Geometry: final body of the model. Coordinates: model frame, mm. Round coordinates to 2 decimals unless told otherwise and drop trailing zeros. Loops run counter-clockwise (first coordinate to the right, second up) from the corner with the lowest first, then second, coordinate; pieces in that order, holes last. Notation, with made-up numbers: (-30.5, 29.25) - (26.5, 29.25) arc R20 ccw to (26.5, 47.25) - close; hole circle Ø11 at (18, 40). An arc over 180 degrees is marked (long way). Answer as a JSON object with one key per item and string values. Group by question number.
Item 1: Section C-C (z = 1). Count the separate pieces of the cut face and the enclosed holes in it, plus the area to 3 significant figures.
Item 2: First-contact query: pin 1 (2.5 mm diameter, centred on x = 35.47, y = 25.41, fed in from -Z); pin 2 (12 mm diameter, centred on x = 11, y = -12.5, fed in from -Z). Flat tips, straight axial feed; report the tip coordinate or a pass-through.
Item 3: Section A-A (y = 2). Return the cut outline in (x, z).
Item 4: Line query: line 1 (X direction, y = 2, z = 0.7); line 2 (X direction, y = 16.5, z = 0.4); line 3 (Y direction, x = 35, z = 1.45). Output: solid intervals per line, ascending.
Item 5: Section B-B (x = 15.5). Return the cut outline in (y, z), plus the area to 3 significant figures.
```python
from build123d import *

# Parameters (mm, degrees)
SKETCH1_W                        = 39.2
SKETCH1_H                        = 58.746225757
BASE_DEPTH                       = 1.5
FRONT_FILLET_R                   = 5
BOLT_HOLE_CUT_REACH              = 51.194
SKETCH4_R                        = 1.6
BOLT_HEAD_CHAMBER_SIZE           = 1.5
CAMRA_HOLE_REACH                 = 51.194
SKETCH2_W                        = 23
SKETCH2_H                        = 21
SKETCH2_W_2                      = 1.25
SKETCH2_H_2                      = 3
SKETCH2_H_3                      = 8
SKETCH9_W                        = 1.5
SKETCH9_H                        = 3
CAMERA_SIDE_MOUNT_HOLDER_DEPTH   = 1.5
FILLET1_R                        = 1
SKETCH12_W                       = 20.06
SKETCH12_H                       = 7.149851194
ANTENNA_CONNECTOR_TOP_BASE_DEPTH = 1.5
ANTENNA_CONNECTOR_TOP_CUT_REACH  = 55.424
SKETCH13_R                       = 3.24
ANTENNA_TOP_CONNECTOR_FILLET_R   = 3
FILLET2_R                        = 1


with BuildPart() as part:
    # Sketch1 → Base (new body)
    with BuildSketch(Plane.XY):
        with Locations((19.622719192, 0.281239742)):
            Rectangle(SKETCH1_W, SKETCH1_H)
    extrude(amount=BASE_DEPTH)

    # Front fillet
    front_fillet_edges = [part.edges().sort_by_distance(p)[0] for p in [
        (0.022719192, 29.65435262, 0.75),
        (39.222719192, 29.65435262, 0.75),
    ]]
    fillet(front_fillet_edges, radius=FRONT_FILLET_R)

    # Sketch4 → Bolt hole cut (cut, up to next)
    with BuildSketch(Plane.XY.offset(1.5), mode=Mode.PRIVATE) as bolt_hole_cut_sk1:
        with Locations((34.872719192, -24.79564738)):
            Circle(SKETCH4_R)
    bolt_hole_cut_tool1 = extrude(bolt_hole_cut_sk1.sketch, amount=-BOLT_HOLE_CUT_REACH, mode=Mode.PRIVATE) & part.part
    # Sketch4 → Bolt hole cut (cut, up to next)
    with BuildSketch(Plane.XY.offset(1.5), mode=Mode.PRIVATE) as bolt_hole_cut_sk2:
        with Locations((4.372719192, -24.79564738)):
            Circle(SKETCH4_R)
    bolt_hole_cut_tool2 = extrude(bolt_hole_cut_sk2.sketch, amount=-BOLT_HOLE_CUT_REACH, mode=Mode.PRIVATE) & part.part
    # Sketch4 → Bolt hole cut (cut, up to next)
    with BuildSketch(Plane.XY.offset(1.5), mode=Mode.PRIVATE) as bolt_hole_cut_sk3:
        with Locations((3.772719192, 25.408275669)):
            Circle(SKETCH4_R)
    bolt_hole_cut_tool3 = extrude(bolt_hole_cut_sk3.sketch, amount=-BOLT_HOLE_CUT_REACH, mode=Mode.PRIVATE) & part.part
    # Sketch4 → Bolt hole cut (cut, up to next)
    with BuildSketch(Plane.XY.offset(1.5), mode=Mode.PRIVATE) as bolt_hole_cut_sk4:
        with Locations((35.472719192, 25.408275669)):
            Circle(SKETCH4_R)
    bolt_hole_cut_tool4 = extrude(bolt_hole_cut_sk4.sketch, amount=-BOLT_HOLE_CUT_REACH, mode=Mode.PRIVATE) & part.part
    add(bolt_hole_cut_tool1.solids().sort_by_distance((34.872719, -24.795647, 1.5))[0], mode=Mode.SUBTRACT)
    add(bolt_hole_cut_tool2.solids().sort_by_distance((4.372719, -24.795647, 1.5))[0], mode=Mode.SUBTRACT)
    add(bolt_hole_cut_tool3.solids().sort_by_distance((3.772719, 25.408276, 1.5))[0], mode=Mode.SUBTRACT)
    add(bolt_hole_cut_tool4.solids().sort_by_distance((35.472719, 25.408276, 1.5))[0], mode=Mode.SUBTRACT)

    # Bolt head chamber
    bolt_head_chamber_edges = [part.edges().sort_by_distance(p)[0] for p in [
        (33.272719192, -24.79564738, 1.5),
        (2.772719192, -24.79564738, 1.5),
        (2.172719192, 25.408275669, 1.5),
        (33.872719192, 25.408275669, 1.5),
    ]]
    chamfer(bolt_head_chamber_edges, length=BOLT_HEAD_CHAMBER_SIZE - 0.0001)  # a hair under: the kernel refuses the full size

    # Sketch2 → Camra hole (cut, up to next)
    with BuildSketch(Plane.XY.offset(1.5), mode=Mode.PRIVATE) as camra_hole_sk1:
        with Locations((19.622719192, 16.15435262)):
            Rectangle(SKETCH2_W, SKETCH2_H)
    camra_hole_tool1 = extrude(camra_hole_sk1.sketch, amount=-CAMRA_HOLE_REACH, mode=Mode.PRIVATE) & part.part
    # Sketch2 → Camra hole (cut, up to next)
    with BuildSketch(Plane.XY.offset(1.5), mode=Mode.PRIVATE) as camra_hole_sk2:
        with Locations((7.497719192, 16.15435262)):
            Rectangle(SKETCH2_W_2, SKETCH2_H)
    camra_hole_tool2 = extrude(camra_hole_sk2.sketch, amount=-CAMRA_HOLE_REACH, mode=Mode.PRIVATE) & part.part
    # Sketch2 → Camra hole (cut, up to next)
    with BuildSketch(Plane.XY.offset(1.5), mode=Mode.PRIVATE) as camra_hole_sk3:
        with Locations((31.747719192, 16.15435262)):
            Rectangle(SKETCH2_W_2, SKETCH2_H)
    camra_hole_tool3 = extrude(camra_hole_sk3.sketch, amount=-CAMRA_HOLE_REACH, mode=Mode.PRIVATE) & part.part
    # Sketch2 → Camra hole (cut, up to next)
    with BuildSketch(Plane.XY.offset(1.5), mode=Mode.PRIVATE) as camra_hole_sk4:
        with Locations((19.622719192, 4.15435262)):
            Rectangle(SKETCH2_W, SKETCH2_H_2)
    camra_hole_tool4 = extrude(camra_hole_sk4.sketch, amount=-CAMRA_HOLE_REACH, mode=Mode.PRIVATE) & part.part
    # Sketch2 → Camra hole (cut, up to next)
    with BuildSketch(Plane.XY.offset(1.5), mode=Mode.PRIVATE) as camra_hole_sk5:
        with Locations((19.622719192, -1.34564738)):
            Rectangle(SKETCH2_W, SKETCH2_H_3)
    camra_hole_tool5 = extrude(camra_hole_sk5.sketch, amount=-CAMRA_HOLE_REACH, mode=Mode.PRIVATE) & part.part
    # Sketch2 → Camra hole (cut, up to next)
    with BuildSketch(Plane.XY.offset(1.5), mode=Mode.PRIVATE) as camra_hole_sk6:
        with Locations((19.622719192, 28.15435262)):
            Rectangle(SKETCH2_W, SKETCH2_H_2)
    camra_hole_tool6 = extrude(camra_hole_sk6.sketch, amount=-CAMRA_HOLE_REACH, mode=Mode.PRIVATE) & part.part
    add(camra_hole_tool1.solids().sort_by_distance((19.622719, 16.154353, 1.5))[0], mode=Mode.SUBTRACT)
    add(camra_hole_tool2.solids().sort_by_distance((7.497719, 16.154353, 1.5))[0], mode=Mode.SUBTRACT)
    add(camra_hole_tool3.solids().sort_by_distance((31.747719, 16.154353, 1.5))[0], mode=Mode.SUBTRACT)
    add(camra_hole_tool4.solids().sort_by_distance((19.622719, 4.154353, 1.5))[0], mode=Mode.SUBTRACT)
    add(camra_hole_tool5.solids().sort_by_distance((19.622719, -1.345647, 1.5))[0], mode=Mode.SUBTRACT)
    add(camra_hole_tool6.solids().sort_by_distance((19.622719, 28.154353, 1.5))[0], mode=Mode.SUBTRACT)

    # Sketch9 → Camera side mount holder (add)
    with BuildSketch(Plane.XY.offset(1.5)):
        with Locations((8.872719192, 28.15435262)):
            Rectangle(SKETCH9_W, SKETCH9_H)
        with Locations((30.372719192, 28.15435262)):
            Rectangle(SKETCH9_W, SKETCH9_H)
    extrude(amount=-CAMERA_SIDE_MOUNT_HOLDER_DEPTH)

    # Fillet1
    fillet1_edges = [part.edges().sort_by_distance(p)[0] for p in [
        (32.372719192, 5.65435262, 0.75),
        (6.872719192, 5.65435262, 0.75),
    ]]
    fillet(fillet1_edges, radius=FILLET1_R)

    # Sketch12 → Antenna connector top base (add)
    with BuildSketch(Plane(origin=(0, 0, 0), x_dir=(-1, 0, 0), z_dir=(0, 0, -1))):
        with Locations((-17.022719192, -32.666798734)):
            Rectangle(SKETCH12_W, SKETCH12_H)
    extrude(amount=-ANTENNA_CONNECTOR_TOP_BASE_DEPTH)

    # Sketch13 → Antenna connector top cut (cut, up to next)
    with BuildSketch(Plane.XY.offset(1.5), mode=Mode.PRIVATE) as antenna_connector_top_cut_sk1:
        with Locations((17.022719192, -31.991873137)):
            Circle(SKETCH13_R)
    antenna_connector_top_cut_tool1 = extrude(antenna_connector_top_cut_sk1.sketch, amount=-ANTENNA_CONNECTOR_TOP_CUT_REACH, mode=Mode.PRIVATE) & part.part
    add(antenna_connector_top_cut_tool1.solids().sort_by_distance((17.022719, -31.991873, 1.5))[0], mode=Mode.SUBTRACT)

    # Antenna top connector fillet
    antenna_top_connector_fillet_edges = [part.edges().sort_by_distance(p)[0] for p in [
        (27.052719192, -29.091873137, 0.75),
        (27.052719192, -36.241724331, 0.75),
        (6.992719192, -36.241724331, 0.75),
        (6.992719192, -29.091873137, 0.75),
    ]]
    fillet(antenna_top_connector_fillet_edges, radius=ANTENNA_TOP_CONNECTOR_FILLET_R)

    # Fillet2
    fillet2_edges = [part.edges().sort_by_distance(p)[0] for p in [
        (32.372719192, 26.65435262, 0.75),
        (31.122719192, -5.34564738, 0.75),
        (8.122719192, -5.34564738, 0.75),
        (6.872719192, 26.65435262, 0.75),
    ]]
    fillet(fillet2_edges, radius=FILLET2_R)


solid = part.part
```
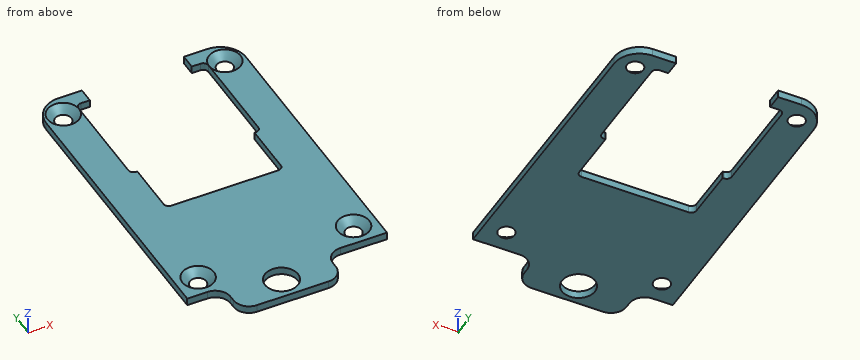
Values:
{
 "1": {"separate pieces": "1", "enclosed holes": "5", "area": "1,470 mm^2"},
 "2": {"pin 1": "passes through", "pin 2": "stops at z = 0"},
 "3": {"outline": "(0.02, 0) - (8.12, 0) - (8.12, 1.5) - (0.02, 1.5) - close; (31.12, 0) - (39.22, 0) - (39.22, 1.5) - (31.12, 1.5) - close"},
 "4": {"line 1": "x = 0.02 to 8.12, 31.12 to 39.22", "line 2": "x = 0.02 to 6.87, 32.37 to 39.22", "line 3": "y = -29.09 to -27.84, -21.75 to 22.4, 28.42 to 29.59"},
 "5": {"outline": "(-36.24, 0) - (-34.85, 0) - (-34.85, 1.5) - (-36.24, 1.5) - close; (-29.13, 0) - (-5.35, 0) - (-5.35, 1.5) - (-29.13, 1.5) - close", "area": "37.8 mm^2"}
}
